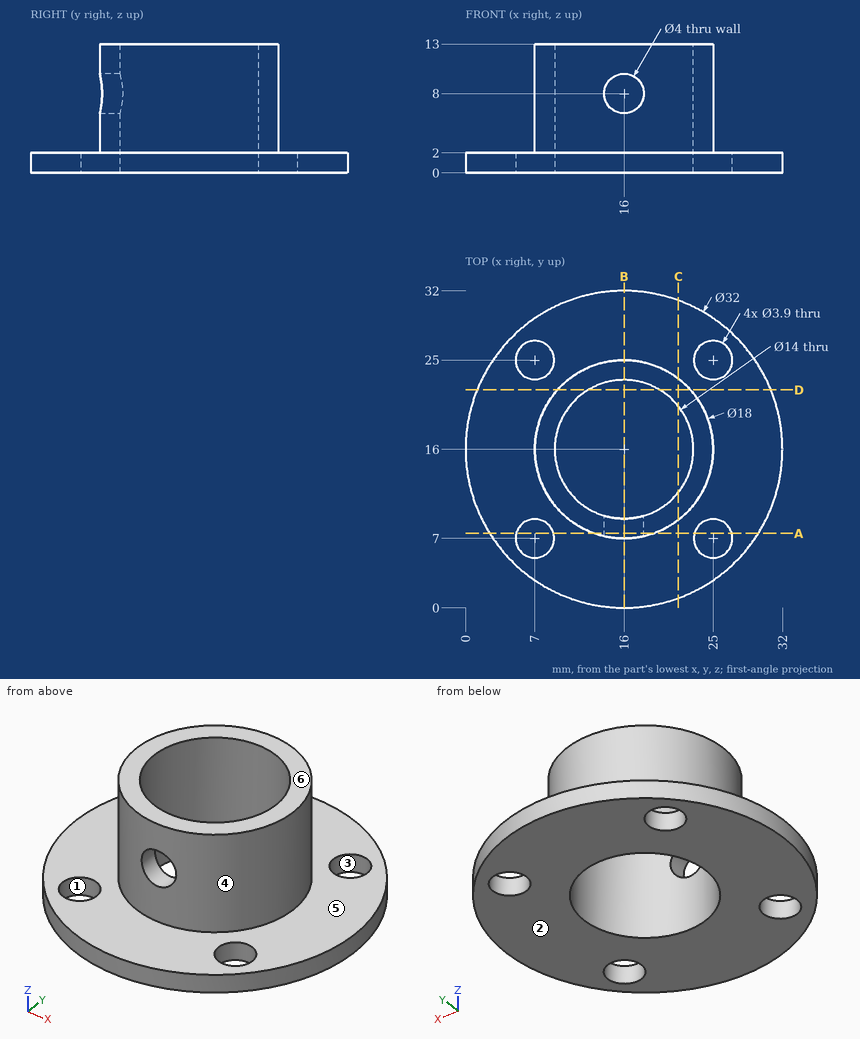
Input: dimensioned drawing with shaded views. Units: mm. Origin: part minimum x, y, z. A direction names the side the tool comes from. Give positions to 0.01 mm unless a question says otherwise; leave off trailing zeros. Loops run counter-clockwise (first coordinate to the right, second up) from the corner with the lowest first, then second, coordinate; pieces in that order, holes last. Notation, with made-up numbers: (-27, 24.5) -> (1, 24.5) arc R32 ccw to (1, 59.5) -> close; hole circle Ø5 at (82.5, 5). An arc over 180 degrees is marked (long way). Return JSON: item names as keys, results as strings.
Item 1: Section D-D, the plane y = 22. Output: boundary loops of the cut face in (x, z), plus the area to 3 significant figures.
Filled in:
{"outline": "(1.17, 0) -> (12.39, 0) -> (12.39, 13) -> (9.29, 13) -> (9.29, 2) -> (1.17, 2) -> close; (19.61, 0) -> (30.83, 0) -> (30.83, 2) -> (22.71, 2) -> (22.71, 13) -> (19.61, 13) -> close", "area": "113 mm^2"}
Item 2: Pin query (flat end, axial travel): P1, Ø2, axis at y = 25, z = 4.5, coming from the -X side; P2, Ø1.5, axis at y = 12, z = 2, coming from the -X side; P3, Ø4.5, axis at x = 16, z = 8, coming from the +Y side. Return the tip coordinate at first contact, or that it passes through.
Filled in:
{"P1": "x = 11.88", "P2": "x = 0.33", "P3": "y = 25"}
Item 3: Section A-A, the plane y = 7.5. Output: boundary loops of the cut face in (x, z), plus the area to 3 significant figures.
Filled in:
{"outline": "(2.44, 0) -> (5.12, 0) -> (5.12, 2) -> (2.44, 2) -> close; (8.88, 0) -> (23.12, 0) -> (23.12, 2) -> (18.96, 2) -> (18.96, 13) -> (13.04, 13) -> (13.04, 2) -> (8.88, 2) -> close; (26.88, 0) -> (29.56, 0) -> (29.56, 2) -> (26.88, 2) -> close; hole circle Ø4 at (16, 8)", "area": "91.7 mm^2"}
Item 4: Section C-C, the plane x = 21.5. Output: boundary loops of the cut face in (y, z), plus the area to 3 significant figures.
Filled in:
{"outline": "(0.98, 0) -> (11.67, 0) -> (11.67, 13) -> (8.88, 13) -> (8.88, 2) -> (0.98, 2) -> close; (20.33, 0) -> (31.02, 0) -> (31.02, 2) -> (23.12, 2) -> (23.12, 13) -> (20.33, 13) -> close", "area": "104 mm^2"}
Item 5: Mould query, pull axis X, two halves, no side actions, for the marked faces 1, 2, 3 and 4. Classes: released by +X, released by -X, zero draft, split by the parting line, or undercut.
Filled in:
{"face 1": "undercut", "face 2": "zero draft", "face 3": "undercut", "face 4": "split by the parting line"}
Item 6: Line query: line 1 (Z direction, x = 16, y = 7.6); line 2 (Y direction, x = 7, z = 0.6); line 3 (Z direction, x = 15, y = 5). Output: solid intervals per line, ascending.
Filled in:
{"line 1": "0 to 6, 10 to 13", "line 2": "2.77 to 5.05, 8.95 to 23.05, 26.95 to 29.23", "line 3": "0 to 2"}
Item 7: Section B-B, the plane x = 16. Output: boundary loops of the cut face in (y, z).
Filled in:
{"outline": "(0, 0) -> (9, 0) -> (9, 6) -> (7, 6) -> (7, 2) -> (0, 2) -> close; (7, 10) -> (9, 10) -> (9, 13) -> (7, 13) -> close; (23, 0) -> (32, 0) -> (32, 2) -> (25, 2) -> (25, 13) -> (23, 13) -> close"}
Item 8: Access query for the marked faces 5 and 6. Directions: +Z, -Z, +X, -X, +Y, -Y. A direction counts if a zero-diameter tool reaches every point of the face in a straight line with its end or side. Return the directions, or none.
Filled in:
{"face 5": "+Z", "face 6": "+Z, +X, -X, +Y, -Y"}
